```python
from build123d import *

# Parameters (mm, degrees)
SKETCH1_W                                           = 44
SKETCH1_H                                           = 27
SKETCH1_R                                           = 8
BOSS_EXTRUDE1_DEPTH                                 = 15
CBORE_FOR_M5_HEX_SOCKET_HEAD_CAP_SCREW1_D           = 5.5
CBORE_FOR_M5_HEX_SOCKET_HEAD_CAP_SCREW1_DEPTH       = 27
CBORE_FOR_M5_HEX_SOCKET_HEAD_CAP_SCREW1_CBORE_D     = 8.5
CBORE_FOR_M5_HEX_SOCKET_HEAD_CAP_SCREW1_CBORE_DEPTH = 6
CHAMFER1_SIZE                                       = 2
CUT_EXTRUDE1_REACH                                  = 17


with BuildPart() as part:
    # Sketch1 → Boss-Extrude1 (new body)
    with BuildSketch(Plane.XY):
        with Locations((0, 13.5)):
            Rectangle(SKETCH1_W, SKETCH1_H)
        with Locations((0, 13)):
            Circle(SKETCH1_R, mode=Mode.SUBTRACT)
    extrude(amount=BOSS_EXTRUDE1_DEPTH)

    # CBORE for M5 Hex Socket Head Cap Screw1
    with Locations(Plane(origin=(-15, 27, 7.5), x_dir=(1, 0, 0), z_dir=(0, 1, 0))):
        with Locations((0, 0), (30, 0)):
            CounterBoreHole(CBORE_FOR_M5_HEX_SOCKET_HEAD_CAP_SCREW1_D / 2, CBORE_FOR_M5_HEX_SOCKET_HEAD_CAP_SCREW1_CBORE_D / 2, CBORE_FOR_M5_HEX_SOCKET_HEAD_CAP_SCREW1_CBORE_DEPTH, depth=CBORE_FOR_M5_HEX_SOCKET_HEAD_CAP_SCREW1_DEPTH)

    # Chamfer1
    chamfer1_edges = [part.edges().sort_by_distance(p)[0] for p in [
        (-22, 27, 7.5),
        (22, 27, 7.5),
    ]]
    chamfer(chamfer1_edges, length=CHAMFER1_SIZE)

    # Sketch4 → Cut-Extrude1 (cut, up to next)
    with BuildSketch(Plane.XY.offset(15), mode=Mode.PRIVATE) as cut_extrude1_sk1:
        with BuildLine():
            Line((7.745966692, 15), (22, 15))
            Line((22, 15), (22, 11))
            Line((22, 11), (7.745966692, 11))
            ThreePointArc((7.745966692, 11), (8, 13), (7.745966692, 15))
        make_face()
    cut_extrude1_tool1 = extrude(cut_extrude1_sk1.sketch, amount=-CUT_EXTRUDE1_REACH, mode=Mode.PRIVATE) & part.part
    add(cut_extrude1_tool1.solids().sort_by_distance((14.957731, 13, 15))[0], mode=Mode.SUBTRACT)


solid = part.part
```
Part model, mm, in its own coordinate system. A direction names the side the tool comes from. Give positions to 0.01 mm unless a question says otherwise; leave off trailing zeros. Write each loop counter-clockwise with the first axis right and the second up, starting at its lowest first coordinate (ties: lowest second). Pieces come first, ordered by that corner, then holes. Notation, with made-up numbers: M 46,52.5 L 92,52.5 A24 ccw 92,86.5 Z; hole C 55,79 d10. An arc over 180 degrees is marked long. Use CSV: the item, a comma, the result in double quotes.
Item 1: Slice it at C-C on x = 15. Write the cut outline in (y, z), plus the area to 4 significant figures.
Taken from the geometry:
outline,"M 0,0 L 11,0 L 11,4.75 L 0,4.75 Z; M 0,10.25 L 11,10.25 L 11,15 L 0,15 Z; M 15,0 L 27,0 L 27,3.25 L 21,3.25 L 21,4.75 L 15,4.75 Z; M 15,10.25 L 21,10.25 L 21,11.75 L 27,11.75 L 27,15 L 15,15 Z"
area,"200.5 mm²"
Item 2: Pin check, flat tips, straight feed: P1, Ø5, axis at x = 15.5, y = 13, coming from the +Z side; P2, Ø7, axis at x = -15, z = 7.5, coming from the +Y side. Stop position of each tip, or through.
Taken from the geometry:
P1,"stops at z = 15"
P2,"stops at y = 21"
Item 3: Slice it at D-D on x = 0. Write the cut outline in (y, z).
Taken from the geometry:
outline,"M 0,0 L 5,0 L 5,15 L 0,15 Z; M 21,0 L 27,0 L 27,15 L 21,15 Z"
Item 4: Drill centre lines: probe 1 along Y at (x, z) = (18.5, 7.5); probe 2 along Z at (x, y) = (-15, 6.25); probe 3 along Y at (x, z) = (17.5, 13.25). Where is each one in solid material? Low to high.
Taken from the geometry:
probe 1,"y = 0 to 11, 15 to 21"
probe 2,"z = 0 to 4.75, 10.25 to 15"
probe 3,"y = 0 to 11, 15 to 27"
Item 5: Pull direction Z, two halves, no side cores. Call faces 1 (the face through (-5, 20, 0)), 2 (the face through (17.182, 17.958, 9.173)), 3 (the face through (21, 26, 7)): +Z half, -Z half, draft (parallel to the pull), parting line (faces both ways), or undercut.
Taken from the geometry:
face 1,"-Z half"
face 2,"undercut"
face 3,"draft"
Item 6: Slice it at A-A on y = 6. Write the cut outline in (x, z).
Taken from the geometry:
outline,"M -22,0 L -3.87,0 L -3.87,15 L -22,15 Z; M 3.87,0 L 22,0 L 22,15 L 3.87,15 Z; hole C -15,7.5 d5.5; hole C 15,7.5 d5.5"
Item 7: Which spindle directions (+Z, -Z, +X, -X, +Y, -Y) get a long thin tool onto all of the face, cutting with end or side? Do faces 4 (the face through (22, 20, 7)), 5 (the face through (18, 15, 8)), 6 (the face through (-13.04, 24.04, 11.27)). Say none if no direction does.
Taken from the geometry:
face 4,"+Z, -Z, +X, +Y, -Y"
face 5,"+Z, -Z, +X"
face 6,"+Y"
Item 8: Slice it at B-B on z = 7.5. State how many separate pieces and enclosed holes the cut face has, plus the area to 3 significant figures.
Taken from the geometry:
separate pieces,"4"
enclosed holes,"0"
area,"616 mm²"
